Can you work these out from the model? Positions are in its coordinate system, mm. A direction names the side the tool comes from. Give positions to 0.01 mm unless a question says otherwise; leave off trailing zeros. Write each loop counter-clockwise with the first axis right and the second up, starting at its lowest first coordinate (ties: lowest second). Pieces come first, ordered by that corner, then holes. Notation, with made-up numbers: (-15, 10) -> (2, 10) arc R27 ccw to (2, 37) -> close; hole circle Ø3 at (-37, 22.25). An arc over 180 degrees is marked (long way). Answer as CSV lines item,"result". Start each with the question number.
1. If we section it at A-A on x = 135: Write out the boundary of the cut face in (y, z).
2. On a 3-axis mill with a long thin cutter (end or side, diameter ignored), from which of +Z, -Z, +X, -X, +Y, -Y can I reach the whole of each face in a straight line? I mean faces 4 (the face through (148, -141, 25)), 5 (the face through (-10, 0, 85)), 6 (the face through (310, 0, 85)). Say none if no direction works.
3. If we mould it in two halves opening along Z, with no side actions, what happens to faces 1 (the face through (147.62, 19.524, 45.664)), 2 (the face through (152, -95, 100)), 3 (the face through (36.023, -98.972, 82.633))? For each: pulls with the +Z half, pulls with the -Z half, needs draft (parallel to the pull), parting line crosses it, or undercut.
4. I'm going to push flat-ended pins straight in: P1, Ø6, axis at x = 309.5, z = 10, coming from the -Y side; P2, Ø5, axis at x = 40, z = 34.5, coming from the +Y side; P3, Ø25, axis at x = 142, z = 53.5, coming from the -Y side. Where does each tip first touch, or does it pass through?
5. If we section it at C-C on y = -200: Write out the boundary of the cut face in (x, z), plus the area to 3 significant figures.
6. I need wall thicknesses on line 1 (Y direction, x = 202.5, z = 50); line 2 (Z direction, x = 161, y = -89.5); line 3 (Y direction, x = 204, z = 51.5). Which ranges of each line are inside material? Lowest first, please. Write a range as [from, to].
7. If we section it at D-D on z = 45: Write out the boundary of the cut face in (x, y), plus the area to 3 significant figures.
8. If we section it at B-B on z = 17.5: Write out the boundary of the cut face in (x, y).
```python
from build123d import *

# Parameters (mm, degrees)
BOSS_EXTRUDE1_DEPTH      = 100
BOSS_EXTRUDE2_DEPTH      = 320
BOSS_EXTRUDE2_DEPTH_BACK = 20
SKETCH3_R                = 20
CUT_EXTRUDE1_DEPTH       = 419.210473327
CUT_EXTRUDE1_DEPTH_BACK  = 419.210473327
SKETCH3_3_R              = 20
CUT_EXTRUDE2_DEPTH       = 419.210473327
CUT_EXTRUDE2_DEPTH_BACK  = 419.210473327
SKETCH4_W                = 50
SKETCH4_H                = 180
SKETCH5_R                = 25
CUT_EXTRUDE5_DEPTH       = 419.210473327


with BuildPart() as part:
    # Sketch2 → Boss-Extrude1 (new body)
    with BuildSketch(Plane.XY):
        Polygon((0, 0), (300, 0), (209.007441433, -250), (90.992558567, -250), align=None)
    extrude(amount=BOSS_EXTRUDE1_DEPTH)

    # Sketch3 → Boss-Extrude2 (add, two sides: drawn at the far end of the back side and taken through both)
    with BuildSketch(Plane(origin=(0, 0, 0), x_dir=(0, 0, -1), z_dir=(1, 0, 0)).offset(-BOSS_EXTRUDE2_DEPTH_BACK)):
        with BuildLine():
            Line((-30, 0), (0, 0))
            ThreePointArc((0, 0), (-50, 50), (-100, 0))
            Line((-100, 0), (-70, 0))
            ThreePointArc((-70, 0), (-50, 20), (-30, 0))
        make_face()
        with Locations((-50, 0)):
            Circle(SKETCH3_R)
    extrude(amount=BOSS_EXTRUDE2_DEPTH + BOSS_EXTRUDE2_DEPTH_BACK)

    # Sketch3_3 → Cut-Extrude1 (cut, two sides: drawn at the far end of the back side and taken through both)
    with BuildSketch(Plane(origin=(0, 0, 0), x_dir=(0, 0, -1), z_dir=(1, 0, 0)).offset(-CUT_EXTRUDE1_DEPTH_BACK)):
        with Locations(Location((-50, 0, 0), (0, 0, 180))):
            Circle(SKETCH3_3_R)
    extrude(amount=CUT_EXTRUDE1_DEPTH + CUT_EXTRUDE1_DEPTH_BACK, mode=Mode.SUBTRACT)

    # Sketch4 → Cut-Extrude2 (cut, two sides: drawn at the far end of the back side and taken through both)
    with BuildSketch(Plane(origin=(0, 0, 0), x_dir=(0, 0, -1), z_dir=(1, 0, 0)).offset(-CUT_EXTRUDE2_DEPTH_BACK)):
        with Locations((-50, -160)):
            Rectangle(SKETCH4_W, SKETCH4_H)
    extrude(amount=CUT_EXTRUDE2_DEPTH + CUT_EXTRUDE2_DEPTH_BACK, mode=Mode.SUBTRACT)

    # Sketch5 → Cut-Extrude5 (cut, through all)
    with BuildSketch(Plane.XY):
        with Locations(Location((150, -200, 0), (0, 0, 90))):
            Circle(SKETCH5_R)
    extrude(amount=CUT_EXTRUDE5_DEPTH, mode=Mode.SUBTRACT)


solid = part.part
```
Computed values:
1,outline,"(-250, 0) -> (-220, 0) -> (-220, 25) -> (-250, 25) -> close; (-250, 75) -> (-220, 75) -> (-220, 100) -> (-250, 100) -> close; (-180, 0) -> (0, 0) arc R50 ccw to (0, 100) -> (-180, 100) -> (-180, 75) -> (-70, 75) -> (-70, 25) -> (-180, 25) -> close; hole circle Ø40 at (0, 50)"
2,face 4,"+X, -X, -Y"
2,face 5,"+Z, -Z, -X, -Y"
2,face 6,"+Z, -Z, +X, -Y"
3,face 1,"undercut"
3,face 2,"pulls with the +Z half"
3,face 3,"needs draft"
4,P1,"stops at y = 0"
4,P2,"stops at y = 48.28"
4,P3,"stops at y = -70"
5,outline,"(72.79, 0) -> (125, 0) -> (125, 25) -> (72.79, 25) -> close; (72.79, 75) -> (125, 75) -> (125, 100) -> (72.79, 100) -> close; (175, 0) -> (227.21, 0) -> (227.21, 25) -> (175, 25) -> close; (175, 75) -> (227.21, 75) -> (227.21, 100) -> (175, 100) -> close"
5,area,"5,220 mm2"
6,line 1,"y = [-70, -20], [20, 50]"
6,line 2,"z = [0, 25], [75, 100]"
6,line 3,"y = [-70, -19.94], [19.94, 49.98]"
7,outline,"(-20, 19.36) -> (320, 19.36) -> (320, 49.75) -> (-20, 49.75) -> close; (7.05, -19.36) -> (25.48, -70) -> (274.52, -70) -> (292.95, -19.36) -> close"
7,area,"23,900 mm2"
8,outline,"(-20, 0) -> (0, 0) -> (90.99, -250) -> (209.01, -250) -> (300, 0) -> (320, 0) -> (320, 38) -> (-20, 38) -> close; hole circle Ø50 at (150, -200)"
